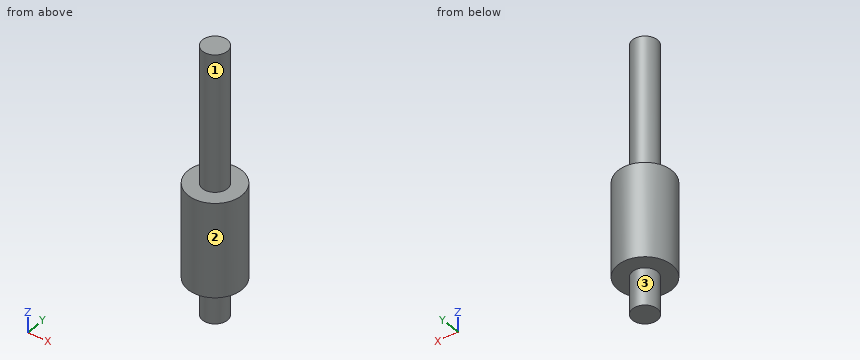
from build123d import *

# Parameters (mm, degrees)
SKETCH1_R           = 6.5
BOSS_EXTRUDE1_DEPTH = 65
CUT_EXTRUDE2_START  = -33.2
SKETCH3_R           = 6.5
SKETCH3_R_2         = 3
CUT_EXTRUDE2_DEPTH  = 33.2
SKETCH4_R           = 6.5
SKETCH4_R_2         = 3
CUT_EXTRUDE3_DEPTH  = 9


with BuildPart() as part:
    # Sketch1 → Boss-Extrude1 (new body)
    with BuildSketch(Plane.XY):
        Circle(SKETCH1_R)
    extrude(amount=BOSS_EXTRUDE1_DEPTH)

    # Sketch3 → Cut-Extrude2 (cut)
    with BuildSketch(Plane.XY.offset(65).offset(CUT_EXTRUDE2_START)):
        Circle(SKETCH3_R)
        Circle(SKETCH3_R_2, mode=Mode.SUBTRACT)
    extrude(amount=CUT_EXTRUDE2_DEPTH, mode=Mode.SUBTRACT)

    # Sketch4 → Cut-Extrude3 (cut)
    with BuildSketch(Plane(origin=(0, 0, 0), x_dir=(-1, 0, 0), z_dir=(0, 0, -1))):
        Circle(SKETCH4_R)
        with Locations(Location((0, 0, 0), (0, 0, 180))):
            Circle(SKETCH4_R_2, mode=Mode.SUBTRACT)
    extrude(amount=-CUT_EXTRUDE3_DEPTH, mode=Mode.SUBTRACT)


solid = part.part
Could you check a few things on this model? Use its own coordinates, in mm. Face numbers are marked on the shaded views. A direction names the side the tool comes from. Coordinates: 2 decimals unless noted, no trailing zeros. Loops run counter-clockwise (first coordinate to the right, second up) from the corner with the lowest first, then second, coordinate; pieces in that order, holes last.
1. For the marked faces 1, 2 and 3, which set-ups out of +Z, -Z, +X, -X, +Y, -Y let a thin tool reach every point of the face, with its end or its side?
2. Imagine slicing it at C-C (z = 45.5). Please give me the cut outline in (x, y).
3. For P1, Ø1.5, axis at y = -2.5, z = 9.5, coming from the -X side; P2, Ø2, axis at x = 3, y = 3.5, coming from the -Z side; P3, Ø6, axis at x = 0, z = 52, coming from the -Y side, each with a flat end and sliding along its axis, tell me the tip position at first contact or that it passes through.
4. Imagine slicing it at A-A (y = 0). Please give me the cut outline in (x, z).
5. I need wall thicknesses on L1, parallel to Z at x = 5.5, y = -3.25; L2, parallel to X at y = -2.5, z = 15; L3, parallel to Y at x = 1, z = 56. Which ranges of each line are inside material? Lowest first, please.
6. Imagine slicing it at D-D (z = 23). Please give me the cut outline in (x, y), and give its area (3 significant figures).
Computed values:
1. face 1: +Z
1. face 2: +Z, -Z
1. face 3: -Z
2. outline: circle Ø6 at (0, 0)
3. P1: stops at x = -6.26
3. P2: stops at z = 9
3. P3: stops at y = -3
4. outline: (-6.5, 9) - (-3, 9) - (-3, 0) - (3, 0) - (3, 9) - (6.5, 9) - (6.5, 31.8) - (3, 31.8) - (3, 65) - (-3, 65) - (-3, 31.8) - (-6.5, 31.8) - close
5. L1: z = 9 to 31.8
5. L2: x = -6 to 6
5. L3: y = -2.83 to 2.83
6. outline: circle Ø13 at (0, 0)
6. area: 133 mm2
